Autodesk Inventor part; units mm, degrees
ref_plane "YZ Plane" through (0, 0, 0) normal (1, 0, 0) x (0, 1, 0)
ref_plane "XZ Plane" through (0, 0, 0) normal (0, 1, 0) x (-1, 0, 0)
ref_plane "XY Plane" through (0, 0, 0) normal (0, 0, 1) x (1, 0, 0)
sketch "Sketch1" plane through (0, 0, 0) normal (0, 1, 0) x (-1, 0, 0)
  line L0 (0, 0) -> (0, -280)
  line L1 (0, -280) -> (17, -280)
  line L2 (17, -280) -> (17, 0)
  line L3 (17, 0) -> (0, 0)
  line L4 (0, 0) -> (-10, 0)
  line L5 (-10, 0) -> (-10, -40)
  line L6 (-10, -40) -> (0, -40)
  line L7 (0, 0) -> (0, -125)
  line L8 (0, 0) -> (-70, 0)
  line L9 (0, -125) -> (0, -145)
  line L10 (0, -145) -> (0, -165)
  line L11 (-70, 0) -> (0, -145)
  circle A0 centre (-70, 0) radius 12.5
  line L12 (-81.2569, -5.4344) -> (0, -173.7522)
  line L13 (-70, 0) -> (-58.7431, 5.4344)
  line L14 (-58.7431, 5.4344) -> (0, -116.2478)
  line L15 (-70, 0) -> (-70, -3.2)
  line L16 (-81.2569, -5.4344) -> (-83.8804, 0)
  line L17 (-64.5656, -11.2569) -> (-64.5656, 0)
  line L18 (-64.5656, 0) -> (-76.5656, 0)
  line L19 (-64.5656, 0) -> (-52.5656, 0)
  line L20 (-64.5656, -11.2569) -> (-64.5656, -19.2569)
  line L21 (-64.5656, -19.2569) -> (-76.5656, -19.2569)
  line L22 (-76.5656, -19.2569) -> (-76.5656, 0)
  line L23 (-64.5656, -19.2569) -> (-52.5656, -19.2569)
  line L24 (-52.5656, -19.2569) -> (-52.5656, 0)
  line L25 (-70, -3.2) -> (-76.5656, -3.2)
  line L26 (-70, -3.2) -> (-52.5656, -3.2)
  line L27 (-52.5656, -3.2) -> (-52.5656, -6.2)
  line L28 (-52.5656, -6.2) -> (-76.5656, -6.2)
  line L29 (-64.5656, -6.2) -> (-64.5656, -12.2)
  circle A1 centre (-64.5656, -12.2) radius 2.4
  line L30 (0, -145) -> (0, -157)
  line L31 (0, -145) -> (0, -133)
  line L32 (0, -145) -> (-3, -145)
  line L33 (-3, -145) -> (-10, -145)
  circle A2 centre (-10, -145) radius 2.25
  line L34 (0, -145) -> (0, -137)
  line L35 (0, -137) -> (-15, -137)
  line L36 (-15, -137) -> (-15, -145)
  line L37 (0, -145) -> (0, -153)
  line L38 (0, -153) -> (-15, -153)
  line L39 (-15, -153) -> (-15, -145)
  line L40 (-3, -145) -> (-3, -137)
  line L41 (-3, -145) -> (-3, -153)
  dimension "d0" = 280
  dimension "d1" = 17
  dimension "d2" = 280
  dimension "d3" = 10
  dimension "d4" = 40
  dimension "d5" = 125
  dimension "d6" = 70
  dimension "d7" = 20
  dimension "d8" = 20
  dimension "d10" = 25
  dimension "d11" = 3.2
  dimension "d12" = 12
  dimension "d13" = 12
  dimension "d14" = 8
  dimension "d16" = 3
  dimension "d17" = 6
  dimension "d18" = 4.8
  dimension "d19" = 12
  dimension "d20" = 12
  dimension "d21" = 3
  dimension "d22" = 7
  dimension "d23" = 4.5
  dimension "d24" = 5
  dimension "d25" = 8
  dimension "d26" = 8
extrude "Extrusion1" add sketch "Sketch1" along normal mid plane 16 contours L0 L11 L40 L35 | L38 L39 L36 L12 | L12 L36 L35 L11 L40 L41 L38 | L32 L40 L11 | L0 L38 L41 L32 | L40 L11 L35
extrude "Extrusion2" cut sketch "Sketch1" along normal mid plane 10 contours L38 L39 L36 L12 | L12 L36 L35 L11 L40 L41 L38 | L40 L11 L35
extrude "Extrusion3" add sketch "Sketch1" along normal mid plane 30 contours L0 L11 L40 L35 | L32 L40 L11 | L0 L38 L41 L32
sketch "Sketch2" plane through (0, -15, -153) normal (-1, 0, 0) x (0, 0, 1)
  line L0 (0, 23) -> (0, 30)
  line L1 (0, 0) -> (0, 30)
  line L2 (0, 30) -> (8, 30)
  line L3 (16, 30) -> (0, 30)
  line L4 (8, 30) -> (8, 27)
  circle A0 centre (8, 27) radius 1.55
  line L5 (0, 0) -> (8, 0)
  line L6 (8, 0) -> (8, 3)
  circle A1 centre (8, 3) radius 1.55
  point P0 (153, 15)
  dimension "d33" = 8
  dimension "d34" = 3
  dimension "d35" = 3.1
  dimension "d36" = 8
  dimension "d37" = 3
  dimension "d38" = 3.1
extrude "Extrusion4" cut sketch "Sketch2" against normal blind 30
fillet "Fillet1" radius 2 4 edges at (1.5, 15, -153) (1.5, -15, -153) (1.5, -15, -137) (1.5, 15, -137)
properties part number "support_clip_base(2)"
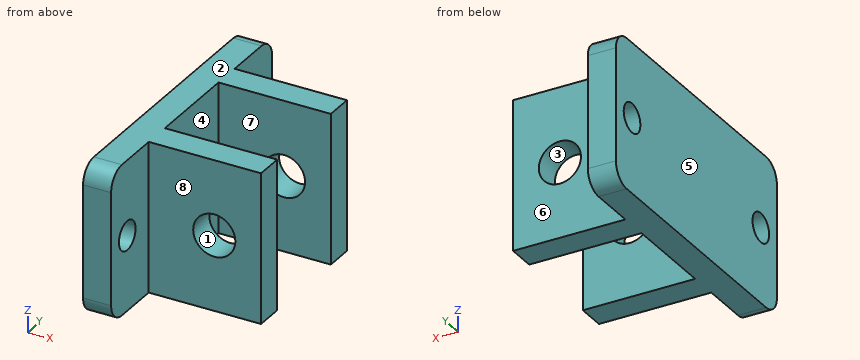
For this review, take the finished solid that the model builds, in its own axes (mm). Face numbers are marked on the shaded views. A direction names the side the tool comes from. Give positions to 0.01 mm unless a question says otherwise; leave off trailing zeros. Write each loop counter-clockwise with the first axis right and the second up, starting at its lowest first coordinate (ties: lowest second). Pieces come first, ordered by that corner, then holes.
Item 1: Take a section at D-D (z = -141). Give the boundary of the cut face in (x, y), and give its area (3 significant figures).
Item 2: The part is to be moulded in two halves that separate along Z. For the marked faces 1, 2, 3 and 4, say which applies: +Z half, -Z half, draft (parallel to the pull), parting line (faces both ways), or undercut.
Item 3: Take a section at B-B (x = 13.5). Give the boundary of the cut face in (y, z).
Item 4: Take a section at C-C (x = 1). Give the boundary of the cut face in (y, z).
Item 5: Take a section at A-A (y = 12). Give the boundary of the cut face in (x, z).
Item 6: Wall thickness on probe 1 along Y at (x, z) = (2.15, -145); probe 2 along Y at (x, z) = (6.25, -139.25); probe 3 along Z at (x, y) = (0.8, -12): over which ranges is each line inside the solid? List them lowest first.
Item 7: Insertion check: P1, Ø2, axis at x = 8.5, z = -148.5, coming from the +Y side; P2, Ø1, axis at y = -0.5, z = -143, coming from the +X side; P3, Ø5, axis at x = 9, y = -1, coming from the +Z side; P4, Ø4, axis at x = 10.5, z = -139, coming from the -Y side. Each pin has a flat end and moves straight along its axis. Give the tip position at first contact, or say it passes through.
Item 8: Machinability: for the marked faces 5, 6, 7 and 8, which of the approach directions +Z, -Z, +X, -X, +Y, -Y give a long, thin tool a straight path to every point of the face, cutting with its end or side? Answer none if there is none.
Established:
1. outline: (0, -15) - (3, -15) - (3, -8) - (15, -8) - (15, -5) - (3, -5) - (3, 5) - (15, 5) - (15, 8) - (3, 8) - (3, 15) - (0, 15) - close
1. area: 162 mm2
2. face 1: undercut
2. face 2: +Z half
2. face 3: undercut
2. face 4: draft
3. outline: (-8, -153) - (-5, -153) - (-5, -137) - (-8, -137) - close; (5, -153) - (8, -153) - (8, -137) - (5, -137) - close
4. outline: (-15, -151) arc R2 ccw to (-13, -153) - (13, -153) arc R2 ccw to (15, -151) - (15, -139) arc R2 ccw to (13, -137) - (-13, -137) arc R2 ccw to (-15, -139) - close; hole circle Ø3.1 at (-12, -145); hole circle Ø3.1 at (12, -145)
5. outline: (0, -153) - (3, -153) - (3, -146.55) - (0, -146.55) - close; (0, -143.45) - (3, -143.45) - (3, -137) - (0, -137) - close
6. probe 1: y = -15 to -13.55, -10.45 to 10.45, 13.55 to 15
6. probe 2: y = -8 to -5, 5 to 8
6. probe 3: z = -153 to -146.55, -143.45 to -137
7. P1: stops at y = 8
7. P2: stops at x = 3
7. P3: passes through
7. P4: stops at y = -8
8. face 5: +Z, -Z, -X, +Y, -Y
8. face 6: +Z, -Z, +X, +Y
8. face 7: +Z, -Z, +X
8. face 8: +Z, -Z, +X, -Y
